from build123d import *

# Parameters (mm, degrees)
F1_W      = 1219.2
F1_H      = 82.55
F2_DEPTH  = 18.2118
F4_DEPTH  = 18.2128
F6_DEPTH  = 18.2128
F7_W      = 38.1
F7_H      = 18.2118
F8_DEPTH  = 18.2118
F9_R      = 5.08
F10_DEPTH = 18.2128


# Not quite as in the source:
# - a variable given as a bare number and used for a length is read in inches; the dataset says mm whatever the document's units were


with BuildPart() as f2:
    # F1 (on Top) → F2 (new body)
    with BuildSketch(Plane.XY):
        Rectangle(F1_W, F1_H)
    extrude(amount=F2_DEPTH)

    # F3 (on face) → F4 (cut, through all)
    with BuildSketch(Plane.XY.offset(18.2118)):
        Polygon((-609.6, 0), (-609.6, -41.275), (-591.3882, -41.275), (-591.3882, -5.08), (-591.3882, 0), (-596.4682, 0), align=None)
        with BuildLine():
            Line((-591.3882, 0), (-591.3882, -5.08))
            ThreePointArc((-591.3882, -5.08), (-587.7960975516, 3.5921024484), (-596.4682, 0))
            Line((-596.4682, 0), (-591.3882, 0))
        make_face()
        with BuildLine():
            Line((591.3882, 0), (596.4682, 0))
            ThreePointArc((596.4682, 0), (587.7960975516, 3.5921024484), (591.3882, -5.08))
            Line((591.3882, -5.08), (591.3882, 0))
        make_face()
        Polygon((591.3882, -5.08), (591.3882, -41.275), (609.6, -41.275), (609.6, 0), (596.4682, 0), (591.3882, 0), align=None)
    extrude(amount=-F4_DEPTH, mode=Mode.SUBTRACT)

    # F5 (on face) → F6 (cut, through all)
    with BuildSketch(Plane.XY.offset(18.2118)):
        Polygon((-300.24705, 41.275), (-318.45885, 41.275), (-318.45885, 12.954), (-318.45885, 0), (-316.6449271791, 0), (-302.0609728209, 0), (-300.24705, 0), (-300.24705, 12.954), align=None)
        with BuildLine():
            Line((-318.45885, 0), (-318.45885, 12.954))
            ThreePointArc((-318.45885, 12.954), (-324.9990417403, 5.434189976), (-316.6449271791, 0))
            Line((-316.6449271791, 0), (-318.45885, 0))
        make_face()
        with BuildLine():
            ThreePointArc((-302.0609728209, 0), (-293.7068582597, 5.434189976), (-300.24705, 12.954))
            Line((-300.24705, 12.954), (-300.24705, 0))
            Line((-300.24705, 0), (-302.0609728209, 0))
        make_face()
        Polygon((318.45885, 41.275), (300.24705, 41.275), (300.24705, 12.954), (300.24705, 0), (302.0609728208, 0), (316.6449271792, 0), (318.45885, 0), (318.45885, 12.954), align=None)
        with BuildLine():
            Line((300.24705, 0), (300.24705, 12.954))
            ThreePointArc((300.24705, 12.954), (293.7068582597, 5.434189976), (302.0609728208, 0))
            Line((302.0609728208, 0), (300.24705, 0))
        make_face()
        with BuildLine():
            ThreePointArc((316.6449271792, 0), (324.9990417403, 5.434189976), (318.45885, 12.954))
            Line((318.45885, 12.954), (318.45885, 0))
            Line((318.45885, 0), (316.6449271792, 0))
        make_face()
        Polygon((9.1059, 41.275), (-9.1059, 41.275), (-9.1059, 12.954), (-9.1059, 0), (-7.2919771792, 0), (7.2919771792, 0), (9.1059, 0), (9.1059, 12.954), align=None)
        with BuildLine():
            Line((-9.1059, 0), (-9.1059, 12.954))
            ThreePointArc((-9.1059, 12.954), (-15.6460917403, 5.434189976), (-7.2919771792, 0))
            Line((-7.2919771792, 0), (-9.1059, 0))
        make_face()
        with BuildLine():
            ThreePointArc((7.2919771792, 0), (15.6460917403, 5.434189976), (9.1059, 12.954))
            Line((9.1059, 12.954), (9.1059, 0))
            Line((9.1059, 0), (7.2919771792, 0))
        make_face()
    extrude(amount=-F6_DEPTH, mode=Mode.SUBTRACT)

    # F7 (on face) → F8 (join)
    with BuildSketch(Plane(origin=(0, 41.275, 0), x_dir=(-1, 0, 0), z_dir=(0, 1, 0))):
        with Locations((590.55, 9.1059)):
            Rectangle(F7_W, F7_H)
        with Locations((-590.55, 9.1059)):
            Rectangle(F7_W, F7_H)
    extrude(amount=F8_DEPTH)

    # F9 (on face) → F10 (cut, through all)
    with BuildSketch(Plane(origin=(0, 0, 0), x_dir=(1, 0, 0), z_dir=(0, 0, -1))):
        with Locations((571.5, -41.275)):
            Circle(F9_R)
        with Locations((-571.5, -41.275)):
            Circle(F9_R)
    extrude(amount=-F10_DEPTH, mode=Mode.SUBTRACT)


solid = f2.part
Here's how the part is built. I have some questions about the finished solid (model axes, mm). Give positions to 0.01 mm unless a question says otherwise; leave off trailing zeros. Order: outer loops, then holes, each group sorted by start corner. A loop starts at its lowest first (then second) coordinate and runs counter-clockwise, first axis right, second up. Notation, with made-up numbers: (-13, 75.5) -> (4, 75.5) arc R30 cw to (4, 108.5) -> close; hole circle Ø1 at (-4, 78). An arc over 180 degrees is marked (long way). One line per item, written item: value. Start each with the question number.
1. Will these pins go through, and if not, where does the flat tip stop? pin 1 Ø10.5 at (x, z) = (-602, 6.5) entering from -Y; pin 2 Ø1 at (x, z) = (175.5, 13) entering from +Y (3 decimals); pin 3 Ø8 at (x, y) = (300.25, 6.35) entering from +Z; pin 4 Ø3 at (y, z) = (-14.5, 10.5) entering from -X.
2. Imagine slicing it at C-C, the plane y = -24.5. List the corners of the cut face in (x, z) for me, plus the area to 3 significant figures.
3. I need wall thicknesses on probe 1 along X at (y, z) = (24.5, 11); probe 2 along X at (y, z) = (6.35, 6.75); probe 3 along X at (y, z) = (52.5, 6.5). Which ranges of each line are inside material? Lowest first, please. Write a range as from..to.
4. Imagine slicing it at B-B, the plane x = 186.5. List the corners of the cut face in (y, z) for me (3 decimals), plus the area to 3 significant figures.
Values follow:
1. pin 1: stops at y = 0
1. pin 2: stops at y = 41.275
1. pin 3: passes through
1. pin 4: stops at x = -591.39
2. outline: (-591.39, 0) -> (591.39, 0) -> (591.39, 18.21) -> (-591.39, 18.21) -> close
2. area: 21,500 mm2
3. probe 1: x = -609.6..-318.46, -300.25..-9.11, 9.11..300.25, 318.46..609.6
3. probe 2: x = -609.6..-325.06, -293.64..-15.71, 15.71..293.64, 325.06..609.6
3. probe 3: x = -609.6..-571.5, 571.5..609.6
4. outline: (-41.275, 0) -> (41.275, 0) -> (41.275, 18.212) -> (-41.275, 18.212) -> close
4. area: 1,500 mm2
